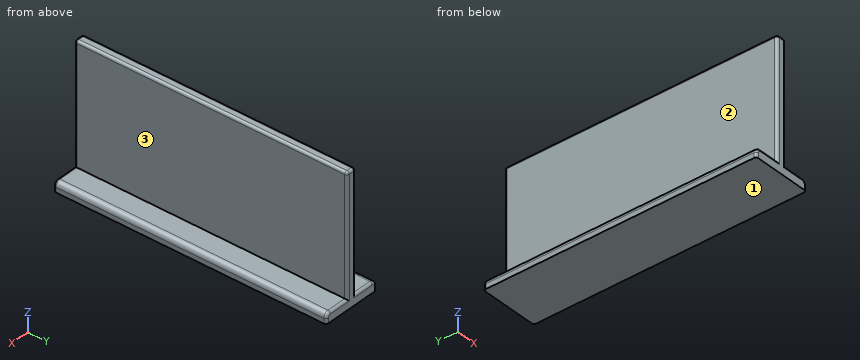
```python
from build123d import *

# Parameters (mm, degrees)
PAD007_DEPTH = 55
FILLET008_R  = 0.5
FILLET009_R  = 1
FILLET010_R  = 0.5
FILLET011_R  = 0.5


with BuildPart() as part:
    # Sketch014 → Pad007 (new body)
    with BuildSketch(Plane.XZ):
        Polygon((0, 0), (12, 0), (12, 2), (7, 2), (7, 26), (5, 26), (5, 2), (0, 2), align=None)
    extrude(amount=PAD007_DEPTH)

    # Fillet008
    fillet008_edges = [part.edges().sort_by_distance(p)[0] for p in [
        (5, -27.5, 26),
        (7, -27.5, 26),
    ]]
    fillet(fillet008_edges, radius=FILLET008_R)

    # Fillet009
    fillet009_edges = [part.edges().sort_by_distance(p)[0] for p in [
        (0, -27.5, 2),
        (12, -27.5, 2),
    ]]
    fillet(fillet009_edges, radius=FILLET009_R)

    # Fillet010
    fillet010_edges = [part.edges().sort_by_distance(p)[0] for p in [
        (5, -55, 13.75),
        (5.146447, -55, 25.853553),
        (6, -55, 26),
        (6.853553, -55, 25.853553),
        (7, -55, 13.75),
        (3, -55, 2),
        (0.292893, -55, 1.707107),
        (0, -55, 0.5),
        (9, -55, 2),
        (11.707107, -55, 1.707107),
        (12, -55, 0.5),
    ]]
    fillet(fillet010_edges, radius=FILLET010_R)

    # Fillet011
    fillet011_edges = [part.edges().sort_by_distance(p)[0] for p in [
        (12, 0, 0.5),
        (11.707107, 0, 1.707107),
        (9, 0, 2),
        (7, 0, 13.75),
        (6.853553, 0, 25.853553),
        (6, 0, 26),
        (5.146447, 0, 25.853553),
        (5, 0, 13.75),
        (3, 0, 2),
        (0.292893, 0, 1.707107),
        (0, 0, 0.5),
    ]]
    fillet(fillet011_edges, radius=FILLET011_R)


with BuildPart() as part_1:
    # Body003 placement: moved
    add(part.part.moved(Location((-45, 55, 0))))


solid = part_1.part
```
For this review, take the finished solid that the model builds, in its own axes (mm). Face numbers are marked on the shaded views. A direction names the side the tool comes from. Coordinates: 2 decimals unless noted, no trailing zeros. Write each loop counter-clockwise with the first axis right and the second up, starting at its lowest first coordinate (ties: lowest second). Pieces come first, ordered by that corner, then holes. Notation, with made-up numbers: (25.25, 83) - (83.25, 83) arc R14 ccw to (83.25, 106) - close; hole circle Ø3 at (-38, -39.5). An arc over 180 degrees is marked (long way). Answer in a Markdown table with one row per item. Add a question column.
Q1. We need section A-A, the plane x = -37.25. State the section outline as (y, z) points.
Q2. We need section B-B, the plane z = 2.5. State the section outline as (x, y) points.
Q3. For P1, Ø5, axis at x = -41, y = 33.5, coming from the -Z side; P2, Ø2, axis at x = -35.5, y = 25, coming from the +Z side; P3, Ø2, axis at y = 15.5, z = 7, coming from the -X side; P4, Ø4, axis at y = 17.5, z = 7, coming from the +X side, all flat-tipped, find the tip position at first contact; note any pin that passes through.
Q4. For probe 1 along X at (y, z) = (18, 6.25); probe 2 along Z at (x, y) = (-36.25, 19); probe 3 along Z at (x, y) = (-44.5, 23), list the stretches that pass through material, from the lowest coordinate up.
Q5. Tool access review of the marked faces 1, 2 and 3: name each direction out of +Z, -Z, +X, -X, +Y, -Y from which nothing blocks a thin tool from reaching the whole face with its end or side.
Q6. We need section C-C, the plane y = 31. State the section outline as (x, z) points.
Answer list:
| question | item | result |
|---|---|---|
| 1 | outline | (0, 0) - (55, 0) - (55, 1.5) arc R0.5 ccw to (54.5, 2) - (0.5, 2) arc R0.5 ccw to (0, 1.5) - close |
| 2 | outline | (-40, 0.5) arc R0.5 ccw to (-39.5, 0) - (-38.5, 0) arc R0.5 ccw to (-38, 0.5) - (-38, 54.5) arc R0.5 ccw to (-38.5, 55) - (-39.5, 55) arc R0.5 ccw to (-40, 54.5) - close |
| 3 | P1 | stops at z = 0 |
| 3 | P2 | stops at z = 2 |
| 3 | P3 | stops at x = -40 |
| 3 | P4 | stops at x = -38 |
| 4 | probe 1 | x = -40 to -38 |
| 4 | probe 2 | z = 0 to 2 |
| 4 | probe 3 | z = 0 to 1.87 |
| 5 | face 1 | -Z, +X, -X, +Y, -Y |
| 5 | face 2 | +Z, -X, +Y, -Y |
| 5 | face 3 | +Z, +X, +Y, -Y |
| 6 | outline | (-45, 0) - (-33, 0) - (-33, 1) arc R1 ccw to (-34, 2) - (-38, 2) - (-38, 25.5) arc R0.5 ccw to (-38.5, 26) - (-39.5, 26) arc R0.5 ccw to (-40, 25.5) - (-40, 2) - (-44, 2) arc R1 ccw to (-45, 1) - close |
